from build123d import *

# Parameters (mm, degrees)
BOSS_EXTRUDE1_DEPTH = 0.15
FILLET4_R           = 2.5
SKETCH3_W           = 2
SKETCH3_H           = 0.4
SKETCH3_W_2         = 1.5
CUT_EXTRUDE1_DEPTH  = 19.603494295


with BuildPart() as part:
    # Sketch1 → Boss-Extrude1 (new, symmetric)
    with BuildSketch(Plane.XY):
        Polygon((0, 0), (-10, 0), (-10, 1.5), (-5, 1.5), (-5, 6), (-3, 6), (-3, 8), (-8.5, 8), (-8.5, 7.5), (-10, 7.5), (-10, 8.5), (-11, 8.5), (-11, 10), (-10, 10), (-10, 15), (0, 15), (3, 15), (3, 0), align=None)
    extrude(amount=BOSS_EXTRUDE1_DEPTH, both=True)

    # Fillet4
    fillet4_edges = [part.edges().sort_by_distance(p)[0] for p in [
        (-5, 1.5, 0),
    ]]
    fillet(fillet4_edges, radius=FILLET4_R)

    # Sketch3 → Cut-Extrude1 (cut, through all)
    with BuildSketch(Plane.XY.offset(0.15)):
        with Locations((1, 5.05)):
            Rectangle(SKETCH3_W, SKETCH3_H)
        with Locations((-2.25, 5.05)):
            Rectangle(SKETCH3_W_2, SKETCH3_H)
        with Locations((1, 10.45)):
            Rectangle(SKETCH3_W, SKETCH3_H)
        with Locations((-3.75, 10.45)):
            Rectangle(SKETCH3_W_2, SKETCH3_H)
    extrude(amount=-CUT_EXTRUDE1_DEPTH, mode=Mode.SUBTRACT)


solid = part.part
Build history of the part. All positions in model axes, mm. Coordinates: 2 decimals unless noted, no trailing zeros. Write each loop counter-clockwise with the first axis right and the second up, starting at its lowest first coordinate (ties: lowest second). Pieces come first, ordered by that corner, then holes.
(1) Cut at D-D on x = -2. List the corners of the cut face in (y, z), and give its area (3 significant figures).
(2) Cut at C-C on x = 1.5. List the corners of the cut face in (y, z), and give its area (3 significant figures).
(3) Cut at A-A on x = -8.75. List the corners of the cut face in (y, z), and give its area (3 significant figures).
(4) Cut at B-B on z = -0.05. State how many separate pieces and enclosed holes the cut face has, and give its area (3 significant figures).
(5) Drill centre lines: line 1 (X direction, y = 5, z = 0); line 2 (Y direction, x = 0.25, z = 0.1); line 3 (Y direction, x = -2.5, z = -0.1). Where is each one in solid material? Low to high.
Working result:
1. outline: (0, -0.15) - (4.85, -0.15) - (4.85, 0.15) - (0, 0.15) - close; (5.25, -0.15) - (15, -0.15) - (15, 0.15) - (5.25, 0.15) - close
1. area: 4.38 mm2
2. outline: (0, -0.15) - (4.85, -0.15) - (4.85, 0.15) - (0, 0.15) - close; (5.25, -0.15) - (10.25, -0.15) - (10.25, 0.15) - (5.25, 0.15) - close; (10.65, -0.15) - (15, -0.15) - (15, 0.15) - (10.65, 0.15) - close
2. area: 4.26 mm2
3. outline: (0, -0.15) - (1.5, -0.15) - (1.5, 0.15) - (0, 0.15) - close; (7.5, -0.15) - (15, -0.15) - (15, 0.15) - (7.5, 0.15) - close
3. area: 2.70 mm2
4. separate pieces: 1
4. enclosed holes: 4
4. area: 159 mm2
5. line 1: x = -5 to -3, -1.5 to 0, 2 to 3
5. line 2: y = 0 to 4.85, 5.25 to 10.25, 10.65 to 15
5. line 3: y = 0 to 4.85, 5.25 to 15
